CAD build for the part. Positions are in the model's coordinates, mm. Give positions to 0.01 mm unless a question says otherwise; leave off trailing zeros. Write each loop counter-clockwise with the first axis right and the second up, starting at its lowest first coordinate (ties: lowest second). Pieces come first, ordered by that corner, then holes. Notation, with made-up numbers: (-15, 53) - (41, 53) arc R19 cw to (41, 87) - close; hole circle Ø9 at (63.25, -33). An arc over 180 degrees is marked (long way). Answer as a JSON object with one key per item and string values.
from build123d import *

# Parameters (mm, degrees)
ESQUISSE1_W              = 15
ESQUISSE1_H              = 15
BOSS_EXTRU_1_DEPTH       = 30
ENL_V_MAT_EXTRU_1_DEPTH  = 30
ENL_V_MAT_EXTRU_2_DEPTH  = 30
ENL_V_MAT_EXTRU_3_DEPTH  = 30
ENL_V_MAT_EXTRU_5_DEPTH  = 30
ENL_V_MAT_EXTRU_7_DEPTH  = 30
ENL_V_MAT_EXTRU_8_DEPTH  = 30
ENL_V_MAT_EXTRU_13_DEPTH = 30
ENL_V_MAT_EXTRU_15_DEPTH = 30
ENL_V_MAT_EXTRU_16_DEPTH = 30
ENL_V_MAT_EXTRU_17_DEPTH = 30
ENL_V_MAT_EXTRU_18_DEPTH = 30
ENL_V_MAT_EXTRU_19_DEPTH = 30
ENL_V_MAT_EXTRU_20_DEPTH = 30
ENL_V_MAT_EXTRU_21_DEPTH = 30
ENL_V_MAT_EXTRU_22_DEPTH = 30
ENL_V_MAT_EXTRU_23_DEPTH = 30
ENL_V_MAT_EXTRU_25_DEPTH = 30
ENL_V_MAT_EXTRU_26_DEPTH = 30


with BuildPart() as part:
    # Esquisse1 → Boss.-Extru.1 (new body)
    with BuildSketch(Plane.XY):
        with Locations((7.5, 7.5)):
            Rectangle(ESQUISSE1_W, ESQUISSE1_H)
    extrude(amount=BOSS_EXTRU_1_DEPTH)

    # Esquisse2 → Enlèv. mat.-Extru.1 (cut)
    with BuildSketch(Plane.ZY):
        Polygon((30, 7.5), (17.157208733, 0), (30, 0), align=None)
    extrude(amount=-ENL_V_MAT_EXTRU_1_DEPTH, mode=Mode.SUBTRACT)

    # Esquisse3 → Enlèv. mat.-Extru.2 (cut)
    with BuildSketch(Plane.ZY):
        Polygon((30, 7.5), (28.775513666, 10.065015711), (21.227680677, 15), (30, 15), align=None)
    extrude(amount=-ENL_V_MAT_EXTRU_2_DEPTH, mode=Mode.SUBTRACT)

    # Esquisse4 → Enlèv. mat.-Extru.3 (cut)
    with BuildSketch(Plane.ZY):
        Polygon((8.926273351, 14.031560197), (13.802198678, 15), (0, 15), (0, 5.06907595), (1.662878512, 6.124252415), (3.211780908, 10.370740256), (4.932627015, 14.031560197), align=None)
        Polygon((3.211780908, 1.321204417), (0, 3.148377639), (0, 0), (7.632757812, 0), align=None)
    extrude(amount=-ENL_V_MAT_EXTRU_3_DEPTH, mode=Mode.SUBTRACT)

    # Esquisse5 → Enlèv. mat.-Extru.5 (cut, along a direction that is not the sketch's normal)
    with BuildSketch(Plane(origin=(0, -7.471488968, 4.363238964), x_dir=(-1, 0, 0), z_dir=(0, -0.863533803, 0.504290959))):
        Polygon((-5.951727483, -29.68819628), (-4.385417014, -26.739512451), (-2.316517921, -26.106069571), (-0.765937965, -20.310025776), (-2.831147462, -15.964380335), (-2.523882774, -14.815829705), (0, -14.815829705), (0, -29.68819628), align=None)
    extrude(amount=-ENL_V_MAT_EXTRU_5_DEPTH, dir=(0, -1, 0), mode=Mode.SUBTRACT)

    # Esquisse6 → Enlèv. mat.-Extru.7 (cut)
    with BuildSketch(Plane(origin=(0, 0, 0), x_dir=(-1, 0, 0), z_dir=(0, -1, 0))):
        Polygon((-0.619141534, -13.957767105), (-2.523882774, -17.157208733), (0, -17.157208733), (0, -7.632757812), (-1.718091984, -7.632757812), (-1.06476411, -9.614809502), align=None)
    extrude(amount=-ENL_V_MAT_EXTRU_7_DEPTH, mode=Mode.SUBTRACT)

    # Esquisse8 → Enlèv. mat.-Extru.8 (cut, along a direction that is not the sketch's normal)
    with BuildSketch(Plane(origin=(0, 2.094023155, 0.625796674), x_dir=(1, 0, 0), z_dir=(0, -0.958129282, -0.286335954))):
        Polygon((1.718091984, 7.313168763), (0.628646684, 4.858294572), (1.46050531, 2.698993008), (0, 2.698993008), (0, 7.313168763), align=None)
    extrude(amount=-ENL_V_MAT_EXTRU_8_DEPTH, dir=(0, -1, 0), mode=Mode.SUBTRACT)

    # Esquisse9 → Enlèv. mat.-Extru.13 (cut, along a direction that is not the sketch's normal)
    with BuildSketch(Plane(origin=(0, 2.378568206, 1.353160834), x_dir=(1, 0, 0), z_dir=(0, -0.869189347, -0.494479401))):
        Polygon((9.741570256, -1.177126716), (7.1144792, -1.556807891), (15, -1.556807891), (15, 2.138337382), (14.506645575, 0.943189576), (12.940964542, -0.714733234), align=None)
        Polygon((3.343379322, -0.797445542), (1.46050531, 2.138337382), (0, 2.138337382), (0, -1.556807891), (4.746944503, -1.556807891), align=None)
    extrude(amount=-ENL_V_MAT_EXTRU_13_DEPTH, dir=(0, -1, 0), mode=Mode.SUBTRACT)

    # Esquisse12 → Enlèv. mat.-Extru.15 (cut, along a direction that is not the sketch's normal)
    with BuildSketch(Plane(origin=(0, -7.471488968, 4.363238964), x_dir=(-1, 0, 0), z_dir=(0, -0.863533803, 0.504290959))):
        Polygon((-9.673460517, -29.68819628), (-12.650110774, -26.711546023), (-14.179932039, -24.105910496), (-13.415021407, -19.903610966), (-15, -14.815829705), (-15, -29.68819628), align=None)
    extrude(amount=-ENL_V_MAT_EXTRU_15_DEPTH, dir=(0, -1, 0), mode=Mode.SUBTRACT)

    # Esquisse13 → Enlèv. mat.-Extru.16 (cut)
    with BuildSketch(Plane(origin=(0, 0, 0), x_dir=(-1, 0, 0), z_dir=(0, -1, 0))):
        Polygon((-15, -12.394983272), (-13.060300751, -7.632757812), (-15, -7.632757812), align=None)
    extrude(amount=-ENL_V_MAT_EXTRU_16_DEPTH, mode=Mode.SUBTRACT)

    # Esquisse14 → Enlèv. mat.-Extru.17 (cut, along a direction that is not the sketch's normal)
    with BuildSketch(Plane(origin=(0, 2.094023155, 0.625796674), x_dir=(1, 0, 0), z_dir=(0, -0.958129282, -0.286335954))):
        Polygon((13.060300751, 7.313168763), (12.024477505, 2.698993008), (15, 2.698993008), (15, 7.313168763), align=None)
    extrude(amount=-ENL_V_MAT_EXTRU_17_DEPTH, dir=(0, -1, 0), mode=Mode.SUBTRACT)

    # Esquisse15 → Enlèv. mat.-Extru.18 (cut, along a direction that is not the sketch's normal)
    with BuildSketch(Plane(origin=(0, 2.378568206, 1.353160834), x_dir=(-1, 0, 0), z_dir=(0, -0.869189347, -0.494479401))):
        Polygon((-12.024477505, -2.138337382), (-8.534571531, 1.351568592), (-12.940964542, 0.714733234), (-14.506645575, -0.943189576), (-15, -2.138337382), align=None)
    extrude(amount=-ENL_V_MAT_EXTRU_18_DEPTH, dir=(0, -1, 0), mode=Mode.SUBTRACT)

    # Esquisse16 → Enlèv. mat.-Extru.19 (cut)
    with BuildSketch(Plane(origin=(0, 0, 0), x_dir=(-1, 0, 0), z_dir=(0, 0, -1))):
        Polygon((-15.396052436, 8.861198197), (-9.123900072, 15.526897376), (-16.183146066, 15.526897376), align=None)
    extrude(amount=-ENL_V_MAT_EXTRU_19_DEPTH, mode=Mode.SUBTRACT)

    # Esquisse17 → Enlèv. mat.-Extru.20 (cut)
    with BuildSketch(Plane(origin=(0, 0, 0), x_dir=(-1, 0, 0), z_dir=(0, 0, -1))):
        Polygon((-6.554218331, 15.18646123), (0.669203066, 7.716085255), (0.669203066, 16.0713818), align=None)
    extrude(amount=-ENL_V_MAT_EXTRU_20_DEPTH, mode=Mode.SUBTRACT)

    # Esquisse18 → Enlèv. mat.-Extru.21 (cut)
    with BuildSketch(Plane(origin=(0, 0, 0), x_dir=(-1, 0, 0), z_dir=(0, 0, -1))):
        Polygon((-15, 9.21839227), (-13.921696564, 6.543051012), (-15.506321771, 4.89668716), (-10.237957447, -0.865586318), (-16.387206956, -0.590246788), (-18.552094895, 8.703903566), (-15.878103341, 10.779733946), align=None)
    extrude(amount=-ENL_V_MAT_EXTRU_21_DEPTH, mode=Mode.SUBTRACT)

    # Esquisse19 → Enlèv. mat.-Extru.22 (cut)
    with BuildSketch(Plane(origin=(0, 0, 0), x_dir=(-1, 0, 0), z_dir=(0, 0, -1))):
        Polygon((-5.875093242, -0.721529481), (0.175293911, 5.616971345), (0.854418999, -0.577472644), (-3.508445206, -1.482972763), align=None)
    extrude(amount=-ENL_V_MAT_EXTRU_22_DEPTH, mode=Mode.SUBTRACT)

    # Esquisse20 → Enlèv. mat.-Extru.23 (cut)
    with BuildSketch(Plane.XZ):
        Polygon((14.641535391, 21.431582068), (7.416422476, 31.42072399), (22.821492514, 29.700662918), (19.193376306, 23.52642454), align=None)
    extrude(amount=-ENL_V_MAT_EXTRU_23_DEPTH, mode=Mode.SUBTRACT)

    # Esquisse21 → Enlèv. mat.-Extru.25 (cut)
    with BuildSketch(Plane(origin=(15, 0, 0), x_dir=(0, 0, -1), z_dir=(1, 0, 0))):
        Polygon((-25.251513547, 13.314322934), (-17.635021909, 15.155835068), (-22.650414381, 16.308069891), (-25.79170864, 15.548569091), align=None)
    extrude(amount=-ENL_V_MAT_EXTRU_25_DEPTH, mode=Mode.SUBTRACT)

    # Esquisse22 → Enlèv. mat.-Extru.26 (cut)
    with BuildSketch(Plane(origin=(0, 0, 0), x_dir=(-1, 0, 0), z_dir=(0, 0, -1))):
        Polygon((-14.178463775, 7.180628802), (-13.430249604, 10.918734357), (-15.892886638, 10.134258582), (-16.358917462, 7.805951421), align=None)
    extrude(amount=-ENL_V_MAT_EXTRU_26_DEPTH, mode=Mode.SUBTRACT)


solid = part.part
Item 1: Cut at B-B (z = 8). Give the cut face in (x, y).
Entries:
{"outline": "(1.6, 3.76) - (5.19, 0) - (11.03, 0) - (13.21, 2.38) - (13.21, 11.18) - (10.53, 14.03) - (5.44, 14.03) - (1.6, 10.06) - close"}
Item 2: Mould opens along Z. For faces 1 (the flat face through (7.24, 8.76, 29.4)), 2 (the flat face through (14.019, 6.118, 19.877)), 3 (the flat face through (1.277, 7.148, 6.68)), 4 (the flat face through (2.935, 2.359, 12.46)) say: +Z half, -Z half, draft (parallel to the pull), parting line (faces both ways), or undercut.
Entries:
{"face 1": "+Z half", "face 2": "undercut", "face 3": "undercut", "face 4": "draft"}
Item 3: Cut at D-D (z = 26). Give the cut face in (x, y).
Entries:
{"outline": "(2.04, 5.16) - (11.34, 5.16) - (11.34, 11.88) - (3.36, 11.88) - (2.04, 10.51) - close"}
Item 4: Probe line 1 (Y direction, x = 8.25, z = 12); line 2 (Y direction, x = 7, z = 4.5); line 3 (Z direction, x = 9.5, y = 5.25). List the from-to ranges inside material, lowest first. Write a range as from..to.
Entries:
{"line 1": "0..14.64", "line 2": "0.94..13.11", "line 3": "1.02..26.15"}
Item 5: Flat gauge pins, fed straight in: P1, Ø4, axis at y = 7.5, z = 25, coming from the +X side; P2, Ø1.5, axis at y = 12, z = 17.5, coming from the +X side; P3, Ø2, axis at x = 7, z = 6, coming from the +Y side; P4, Ø6, axis at x = 8.5, y = 4.5, coming from the -Z side. Where does each tip first touch, or does it go through?
Entries:
{"P1": "x = 13.51", "P2": "x = 13.15", "P3": "y = 14.03", "P4": "z = 0"}
Item 6: Cut at A-A (x = 8). Give the cut face in (y, z).
Entries:
{"outline": "(0, 7.63) - (1.32, 3.21) - (3.09, 0.11) - (5.14, 0.11) - (6.12, 1.66) - (10.37, 3.21) - (14.03, 4.93) - (14.03, 8.93) - (15, 13.8) - (15, 18.28) - (13.87, 22.96) - (10.07, 28.78) - (7.5, 30) - (0, 17.16) - close"}
Item 7: Cut at C-C (y = 8.25). Give the cut face in (x, z).
Entries:
{"outline": "(0.62, 13.96) - (1.06, 9.61) - (1.72, 7.63) - (0.63, 5.28) - (1.46, 3.21) - (2.03, 2.44) - (11.13, 2.44) - (12.02, 3.21) - (13.06, 7.63) - (13.96, 9.85) - (13.96, 20.03) - (13.42, 21.55) - (13.67, 22.77) - (8.7, 29.64) - (5.73, 29.64) - (4.39, 27.45) - (2.32, 26.91) - (0.77, 21.9) - (2.83, 18.15) - (2.52, 17.16) - close"}
